Here's how the part is built. I have some questions about the finished solid (model axes, mm). A direction names the side the tool comes from. Round coordinates to 2 decimals unless told otherwise and drop trailing zeros. Order: outer loops, then holes, each group sorted by start corner. A loop starts at its lowest first (then second) coordinate and runs counter-clockwise, first axis right, second up. Notation, with made-up numbers: M 24.25,27.5 L 29.25,27.5 A23 cw 29.25,38.5 Z; hole C 83.5,-39 d2. An arc over 180 degrees is marked long. Write item = value, one per line. Start each with the question number.
Item 1: For faces 5 (the face through (-339.44, 9.86, -135.19)), 6 (the face through (-303.786, 150.645, 78.049)), which set-ups out of +Z, -Z, +X, -X, +Y, -Y let a thin tool reach every point of the face, with its end or its side?
Item 2: Please list where these lines run through material, in increasing order: L1, parallel to X at y = 15, z = -125.98; L2, parallel to X at y = 14, z = 113; L3, parallel to Y at x = -40.5, z = 41.
Item 3: I'm going to push flat-ended pins straight in: P1, Ø2, axis at x = -312, z = -26, coming from the -Y side; P2, Ø8, axis at x = -55.5, z = 36.5, coming from the +Y side. Where does each tip first touch, or does it pass through?
Item 4: I want a section at A-A, the plane z = 0. List the corners of the cut face in (x, y) for me, plus the area to 3 significant figures.
Item 5: I want a section at C-C, the plane y = 115.5. List the corners of the cut face in (x, z) for me, plus the area to 3 significant figures.
Item 6: I want a section at B-B, the plane x = -295. List the corners of the cut face in (y, z) for me, plus the area to 3 significant figures.
Item 7: We'd pull the mould along Z, two halves only. Please class faces 1 (the face through (-303.786, 150.645, -81.951)), 2 (the face through (-169, 10, -175)), 3 (the face through (-295, 285, 80)), 4 (the face through (-11.59, 9.86, -15.12)): pulls with the +Z half, pulls with the -Z half, needs draft (parallel to the pull), parting line crosses it, or undercut.
Item 8: I want a section at D-D, the plane z = -80. List the corners of the cut face in (x, y) for me, plus the area to 3 significant figures.
```python
from build123d import *

# Parameters (mm, degrees)
SKETCH1_W           = 510
SKETCH1_H           = 350
SKETCH1_R           = 19.05
SKETCH1_R_2         = 12.5
BOSS_EXTRUDE1_DEPTH = 20
SKETCH3_R           = 9
BOSS_EXTRUDE2_DEPTH = 265


with BuildPart() as part:
    # Sketch1 → Boss-Extrude1 (new body)
    with BuildSketch(Plane(origin=(0, 0, 0), x_dir=(1, 0, 0), z_dir=(0, 1, 0))):
        with Locations((-165, 0)):
            Rectangle(SKETCH1_W, SKETCH1_H)
        with Locations(Location((0, 0, 0), (0, 0, 270))):
            Circle(SKETCH1_R, mode=Mode.SUBTRACT)
        with Locations(Location((-347.89, 125.98, 0), (0, 0, 270))):
            Circle(SKETCH1_R_2, mode=Mode.SUBTRACT)
        with Locations(Location((-352, -113.99, 0), (0, 0, 270))):
            Circle(SKETCH1_R_2, mode=Mode.SUBTRACT)
    extrude(amount=BOSS_EXTRUDE1_DEPTH)

    # Sketch3 → Boss-Extrude2 (add)
    with BuildSketch(Plane(origin=(0, 20, 0), x_dir=(1, 0, 0), z_dir=(0, 1, 0))):
        with Locations(Location((-295, 80, 0), (0, 0, 270))):
            Circle(SKETCH3_R)
        with Locations(Location((-295, -80, 0), (0, 0, 270))):
            Circle(SKETCH3_R)
    extrude(amount=BOSS_EXTRUDE2_DEPTH)


solid = part.part
```
Filled in:
q1.face_5 = +Y, -Y
q1.face_6 = +Y
q2.L1 = -420 to -360.39, -335.39 to 90
q2.L2 = -420 to -364.46, -339.54 to 90
q2.L3 = 0 to 20
q3.P1 = 0
q3.P2 = 20
q4.outline = M -420,0 L -19.05,0 L -19.05,20 L -420,20 Z; M 19.05,0 L 90,0 L 90,20 L 19.05,20 Z
q4.area = 9,440 mm^2
q5.outline = C -295,-80 d18; C -295,80 d18
q5.area = 509 mm^2
q6.outline = M 0,-175 L 20,-175 L 20,-89 L 285,-89 L 285,-71 L 20,-71 L 20,71 L 285,71 L 285,89 L 20,89 L 20,175 L 0,175 Z
q6.area = 16,500 mm^2
q7.face_1 = undercut
q7.face_2 = pulls with the -Z half
q7.face_3 = needs draft
q7.face_4 = undercut
q8.outline = M -420,0 L 90,0 L 90,20 L -286,20 L -286,285 L -304,285 L -304,20 L -420,20 Z
q8.area = 15,000 mm^2
